from build123d import *

# Parameters (mm, degrees)
F0_W     = 100
F0_H     = 70
F1_DEPTH = 115
F3_DEPTH = 110
F4_R     = 7.5
F5_DEPTH = 25
F6_SIZE  = 3
F7_SIZE  = 5


with BuildPart() as f1:
    # F0 (on Top) → F1 (new body)
    with BuildSketch(Plane.XY):
        with Locations((50, 35)):
            Rectangle(F0_W, F0_H)
    extrude(amount=F1_DEPTH)

    # F2 (on face) → F3 (cut)
    with BuildSketch(Plane.XY.offset(115)):
        Polygon((20.5, 60), (10, 60), (10, 50.309684), (20.5, 50.309684), (20.5, 55.5), align=None)
        Polygon((90, 60), (79.5, 60), (79.5, 55.5), (79.5, 51), (90, 51), align=None)
        Polygon((20.5, 19), (10, 19), (10, 10), (20.5, 10), (20.5, 14.5), align=None)
        Polygon((90, 10), (90, 19.087384), (79.5, 19.087384), (79.5, 14.5), (79.5, 10), align=None)
        Polygon((20.5, 50.309684), (10, 50.309684), (10, 19), (20.5, 19), (20.5, 14.5), (79.5, 14.5), (79.5, 19.087384), (90, 19.087384), (90, 51), (79.5, 51), (79.5, 55.5), (20.5, 55.5), align=None)
    extrude(amount=-F3_DEPTH, mode=Mode.SUBTRACT)

    # F4 (on face) → F5 (cut)
    with BuildSketch(Plane.XY.offset(5)):
        with Locations((50, 35)):
            Circle(F4_R)
    extrude(amount=-F5_DEPTH, mode=Mode.SUBTRACT)

    # F6
    f6_edges = [f1.edges().sort_by_distance(p)[0] for p in [
        (42.5, 35, 5),
    ]]
    chamfer(f6_edges, length=F6_SIZE)

    # F7
    f7_edges = [f1.edges().sort_by_distance(p)[0] for p in [
        (0, 35, 115),
        (50, 0, 115),
        (100, 35, 115),
        (50, 70, 115),
        (100, 0, 57.5),
        (100, 70, 57.5),
        (0, 70, 57.5),
        (0, 0, 57.5),
    ]]
    chamfer(f7_edges, length=F7_SIZE)


solid = f1.part
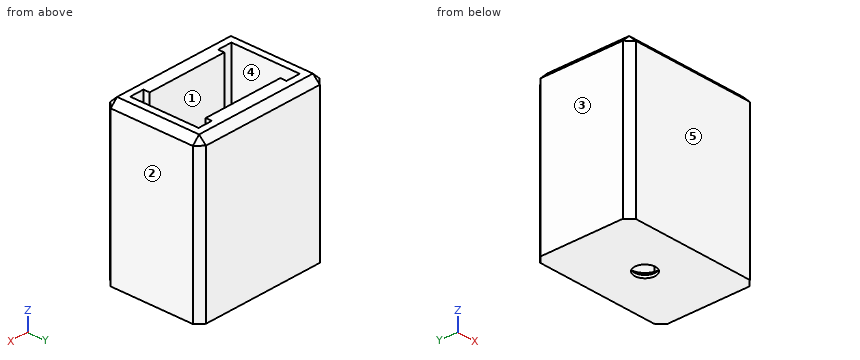
Could you check a few things on this model? Use its own coordinates, in mm. Face numbers are marked on the shaded views. A direction names the side the tool comes from. Coordinates: 2 decimals unless noted, no trailing zeros. Loops run counter-clockwise (first coordinate to the right, second up) from the corner with the lowest first, then second, coordinate; pieces in that order, holes last.
1. Imagine slicing it at A-A (y = 35). Please give me the cut outline in (x, z), and give its area (3 significant figures).
2. Imagine slicing it at B-B (x = 50). Please give me the cut outline in (y, z).
3. Imagine slicing it at C-C (z = 107). Please give me the cut outline in (x, y), and give its area (3 significant figures).
4. We'd pull the mould along X, two halves only. Please class the marked faces 3, 4 and 5: released by +X, released by -X, zero draft, split by the parting line, or undercut.
5. For the marked faces 1 and 2, which set-ups out of +Z, -Z, +X, -X, +Y, -Y let a thin tool reach every point of the face, with its end or its side?
6. I need wall thicknesses on L1, parallel to X at y = 11.5, z = 46; L2, parallel to Y at x = 50, z = 1.2; L3, parallel to X at y = 43, z = 67. Which ranges of each line are inside material? Lowest first, please.
7. For P1, Ø5, axis at x = 86.5, y = 50.5, coming from the +Z side, with a flat end and sliding along its axis, tell me the tip position at first contact or that it passes through.
8. Imagine slicing it at D-D (x = 87.5). Please give me the cut outline in (y, z).
Computed values:
1. outline: (0, 0) - (42.5, 0) - (42.5, 2) - (39.5, 5) - (10, 5) - (10, 115) - (5, 115) - (0, 110) - close; (57.5, 0) - (100, 0) - (100, 110) - (95, 115) - (90, 115) - (90, 5) - (60.5, 5) - (57.5, 2) - close
1. area: 2,590 mm2
2. outline: (0, 0) - (27.5, 0) - (27.5, 2) - (24.5, 5) - (14.5, 5) - (14.5, 115) - (5, 115) - (0, 110) - close; (42.5, 0) - (70, 0) - (70, 110) - (65, 115) - (55.5, 115) - (55.5, 5) - (45.5, 5) - (42.5, 2) - close
3. outline: (0, 5) - (5, 0) - (95, 0) - (100, 5) - (100, 65) - (95, 70) - (5, 70) - (0, 65) - close; hole (10, 10) - (20.5, 10) - (20.5, 14.5) - (79.5, 14.5) - (79.5, 10) - (90, 10) - (90, 60) - (79.5, 60) - (79.5, 55.5) - (20.5, 55.5) - (20.5, 60) - (10, 60) - close
3. area: 3,480 mm2
4. face 3: released by -X
4. face 4: undercut
4. face 5: zero draft
5. face 1: +Z
5. face 2: +Z, -Z, +X, +Y, -Y
6. L1: x = 0 to 10, 20.5 to 79.5, 90 to 100
6. L2: y = 0 to 27.5, 42.5 to 70
6. L3: x = 0 to 10, 90 to 100
7. P1: stops at z = 5
8. outline: (0, 0) - (70, 0) - (70, 110) - (65, 115) - (60, 115) - (60, 5) - (10, 5) - (10, 115) - (5, 115) - (0, 110) - close
